Check sheet for the drawn part. Datum: minimum x, y, z corner. Units: mm. A direction names the side the tool comes from. Round coordinates to 2 decimals unless told otherwise and drop trailing zeros. Order: outer loops, then holes, each group sorted by start corner. A loop starts at its lowest first (then second) coordinate and runs counter-clockwise, first axis right, second up.
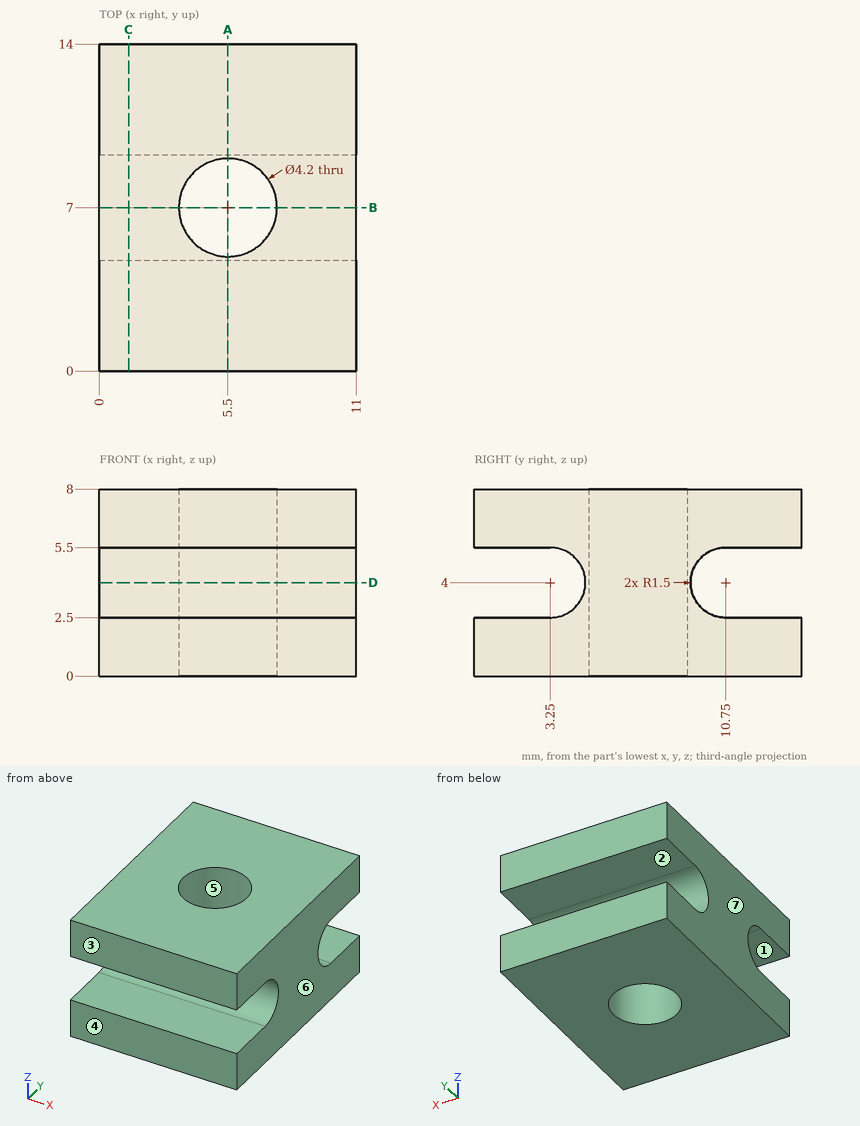
(1) Set-up check for the marked faces 1, 2 and 3: record each of +Z, -Z, +X, -X, +Y, -Y from which the full face is reachable in a straight line by a thin tool's end or side.
Returned:
face 1: +X, -X, -Y
face 2: +X, -X, +Y
face 3: +Z, -Z, +X, -X, -Y
(2) Draft check along X on the marked faces 4, 5, 6 and 7. Enter one of: released by +X, released by -X, zero draft, split by the parting line, or undercut.
Returned:
face 4: zero draft
face 5: undercut
face 6: released by +X
face 7: released by -X
(3) Sectioned sample at C-C, the plane x = 1.25. Record the cut outline in (y, z).
Returned:
outline: (0, 0) - (14, 0) - (14, 2.5) - (10.75, 2.5) arc R1.5 cw to (10.75, 5.5) - (14, 5.5) - (14, 8) - (0, 8) - (0, 5.5) - (3.25, 5.5) arc R1.5 cw to (3.25, 2.5) - (0, 2.5) - close
(4) Sectioned sample at D-D, the plane z = 4. Record the cut outline in (x, y), and give its area (3 significant figures).
Returned:
outline: (0, 4.75) - (11, 4.75) - (11, 9.25) - (0, 9.25) - close; hole circle Ø4.2 at (5.5, 7)
area: 35.6 mm2
(5) Sectioned sample at B-B, the plane y = 7. Record the cut outline in (x, z), and give its area (3 significant figures).
Returned:
outline: (0, 0) - (3.4, 0) - (3.4, 8) - (0, 8) - close; (7.6, 0) - (11, 0) - (11, 8) - (7.6, 8) - close
area: 54.4 mm2
(6) Material ranges on line 1 (Z direction, x = 5.5, y = 11.75); line 2 (Y direction, x = 5.5, z = 6.5); line 3 (Y direction, x = 5.5, z = 3), recorded low to high.
Returned:
line 1: z = 0 to 2.5, 5.5 to 8
line 2: y = 0 to 4.9, 9.1 to 14
line 3: y = 4.37 to 4.9, 9.1 to 9.63
(7) Depth check by flat-ended pin: P1, Ø5.5, axis at x = 5.5, y = 7, coming from the -Z side. Enter the tip coordinate at first touch or a pass-through.
Returned:
P1: stops at z = 0
(8) Sectioned sample at A-A, the plane x = 5.5. Record the cut outline in (y, z).
Returned:
outline: (0, 0) - (4.9, 0) - (4.9, 8) - (0, 8) - (0, 5.5) - (3.25, 5.5) arc R1.5 cw to (3.25, 2.5) - (0, 2.5) - close; (9.1, 0) - (14, 0) - (14, 2.5) - (10.75, 2.5) arc R1.5 cw to (10.75, 5.5) - (14, 5.5) - (14, 8) - (9.1, 8) - close
